from build123d import *

# Parameters (mm, degrees)
F0_R     = 12.5
F0_R_2   = 6
F1_DEPTH = 25
F2_R     = 12.5
F2_R_2   = 6
F3_DEPTH = 12.5
F5_R     = 7.5
F7_DEPTH = 25.0010001
F8_DEPTH = 25


with BuildPart() as f1:
    # F0 (on Front) → F1 (new body)
    with BuildSketch(Plane.XZ):
        Circle(F0_R)
        Circle(F0_R_2, mode=Mode.SUBTRACT)
    extrude(amount=-F1_DEPTH)



with BuildPart() as f3:
    # F2 (on Front) → F3 (new body, symmetric)
    with BuildSketch(Plane.XZ):
        with Locations((150, 0)):
            Circle(F2_R)
        with Locations((150, 0)):
            Circle(F2_R_2, mode=Mode.SUBTRACT)
    extrude(amount=F3_DEPTH, both=True)


with BuildPart() as f1_1:
    add(f1.part)

    add(f3.part)  # F6 merges F3
    # F6: sweep along a path in F4
    with BuildLine(Plane.XY) as f6_path:
        Line((0, 12), (25, 12))
        ThreePointArc((25, 12), (32.1487132371, 11.5726103092), (39.1955835962, 10.2965299685))
        ThreePointArc((39.1955835962, 10.2965299685), (81.789999989, 2.5833332421), (125, 0))
        Line((125, 0), (150, 0))
    # F5 (on Right) → F6 (sweep)
    with BuildSketch(Plane.YZ):
        with Locations((12.4965049244, 0)):
            Circle(F5_R)
    sweep(path=f6_path.line)

    # F0 (on Front) → F7 (cut, through all)
    with BuildSketch(Plane.XZ):
        Circle(F0_R_2)
    extrude(amount=-F7_DEPTH, mode=Mode.SUBTRACT)

    # F2 (on Front) → F8 (cut, symmetric)
    with BuildSketch(Plane.XZ):
        with Locations((150, 0)):
            Circle(F2_R_2)
    extrude(amount=F8_DEPTH, both=True, mode=Mode.SUBTRACT)


solid = f1_1.part
Design review of the part built by this model. Coordinates are the model's own, in mm. A direction names the side the tool comes from. Give positions to 0.01 mm unless a question says otherwise; leave off trailing zeros. Order: outer loops, then holes, each group sorted by start corner. A loop starts at its lowest first (then second) coordinate and runs counter-clockwise, first axis right, second up. Notation, with made-up numbers: (-3, 9.5) - (45, 9.5) arc R28 ccw to (45, 42.5) - close; hole circle Ø7 at (48, -15). An arc over 180 degrees is marked (long way). Use CSV: the item, a comma, the result in double quotes. Start each with the question number.
Q1. Take a section at D-D (x = 17.5). State the section outline as (y, z) points.
Q2. For P1, Ø4, axis at x = 30, y = 12, coming from the -Z side; P2, Ø12, axis at y = -4.5, z = -7, coming from the -X side; P3, Ø3, axis at x = 19.5, z = 9.5, coming from the +Y side; P4, Ø1, axis at x = 43, z = 6.5, coming from the +Y side, all flat-tipped, find the tip position at first contact; note any pin that passes through.
Q3. Take a section at A-A (z = 0). State the section outline as (x, y) points.
Q4. Take a section at B-B (x = 150). State the section outline as (y, z) points.
Q5. Machinability: for faces 1 (the face through (155.4, 12.5, 3)), 2 (the face through (-6, 12, 0)), 3 (the face through (17.605, 19.425, -2.873)), which of the approach directions +Z, -Z, +X, -X, +Y, -Y give a long, thin tool a straight path to every point of the face, cutting with its end or side? Answer none if there is none.
Q6. For line 1 (Z direction, x = 0, y = 11); line 2 (Y direction, x = 151, z = 7); line 3 (Z direction, x = 60, y = 6), list the stretches that pass through material, from the lowest coordinate up.
Q7. Take a section at C-C (z = -11). State the section outline as (x, y) points, and give its area (3 significant figures).
Q8. Draft analysis for pull direction Z (two halves, no side actions). For faces 4 (the face through (161.923, -0.175, 3.755)), 5 (the face through (145.24, 0.18, -3.65)), 6 (the face through (-3, 0, -5.4)), state which applies: pulls with the +Z half, pulls with the -Z half, needs draft (parallel to the pull), parting line crosses it, or undercut.
Calculated:
1,outline,"circle Ø15 at (12.5, 0)"
2,P1,"stops at z = -7.5"
2,P2,"stops at x = -12.13"
2,P3,"passes through"
2,P4,"stops at y = 14.53"
3,outline,"(-12.5, 0) - (-6, 0) - (-6, 25) - (-12.5, 25) - close; (6, 0) - (12.5, 0) - (12.5, 5) - (25, 5) arc R53 cw to (37.54, 3.49) arc R369.67 ccw to (125, -7) - (137.5, -7) - (137.5, -12.5) - (144, -12.5) - (144, 12.5) - (137.5, 12.5) - (137.5, 8) - (125, 8) arc R354.67 cw to (41.09, 18.07) arc R68 ccw to (25, 20) - (12.5, 20) - (12.5, 25) - (6, 25) - close; (156, -12.5) - (162.5, -12.5) - (162.5, 12.5) - (156, 12.5) - close"
4,outline,"(-12.5, -12.5) - (12.5, -12.5) - (12.5, -6) - (-12.5, -6) - close; (-12.5, 6) - (12.5, 6) - (12.5, 12.5) - (-12.5, 12.5) - close"
5,face 1,"+Z, -Z, +X, +Y"
5,face 2,"+Y, -Y"
5,face 3,"none"
6,line 1,"z = -12.5 to -6, 6 to 12.5"
6,line 2,"y = -12.5 to 12.5"
6,line 3,"z = -7.49 to 7.49"
7,outline,"(-5.94, 0) - (5.94, 0) - (5.94, 25) - (-5.94, 25) - close; (144.06, -12.5) - (155.94, -12.5) - (155.94, 12.5) - (144.06, 12.5) - close"
7,area,"594 mm²"
8,face 4,"parting line crosses it"
8,face 5,"undercut"
8,face 6,"needs draft"
